```python
from build123d import *

# Parameters (mm, degrees)
SCHIZZO1_W                               = 70
SCHIZZO1_H                               = 100
ESTRUSIONE_ESTRUSIONE1_DEPTH             = 20
FORO_SVASATO_PER_VITE_M3_5_2_D           = 3.9
FORO_SVASATO_PER_VITE_M3_5_2_CSINK_D     = 8.2
FORO_SVASATO_PER_VITE_M3_5_2_CSINK_ANGLE = 90
SCHIZZO8_W                               = 85
SCHIZZO8_H                               = 40
TAGLIO_ESTRUSIONE1_DEPTH                 = 65.226162893
RACCORDO2_R                              = 5


with BuildPart() as part:
    # Schizzo1 → Estrusione-Estrusione1 (new body)
    with BuildSketch(Plane(origin=(0, 0, 0), x_dir=(0, 1, 0), z_dir=(0, 0, 1))):
        Rectangle(SCHIZZO1_W, SCHIZZO1_H)
    extrude(amount=ESTRUSIONE_ESTRUSIONE1_DEPTH)

    # Foro svasato per Vite M3.5-2 (through all)
    with Locations(Plane.XY.offset(20)):
        with Locations((-45, -20), (30, -29)):
            foro_svasato_per_vite_m3_5_2 = CounterSinkHole(FORO_SVASATO_PER_VITE_M3_5_2_D / 2, FORO_SVASATO_PER_VITE_M3_5_2_CSINK_D / 2, counter_sink_angle=FORO_SVASATO_PER_VITE_M3_5_2_CSINK_ANGLE)

    # Specchia1: Foro svasato per Vite M3.5-2 across plane
    add(foro_svasato_per_vite_m3_5_2.mirror(Plane.ZX), mode=Mode.SUBTRACT)

    # Schizzo8 → Taglio-Estrusione1 (cut, through all)
    with BuildSketch(Plane.XY.offset(20)):
        with Locations((7.5, 0)):
            Rectangle(SCHIZZO8_W, SCHIZZO8_H)
    extrude(amount=-TAGLIO_ESTRUSIONE1_DEPTH, mode=Mode.SUBTRACT)

    # Raccordo2
    raccordo2_edges = [part.edges().sort_by_distance(p)[0] for p in [
        (50, 20, 10),
        (50, -20, 10),
        (-35, -20, 10),
        (-35, 20, 10),
        (50, 35, 10),
        (50, -35, 10),
        (-50, -35, 10),
        (-50, 35, 10),
    ]]
    fillet(raccordo2_edges, radius=RACCORDO2_R)


solid = part.part
```
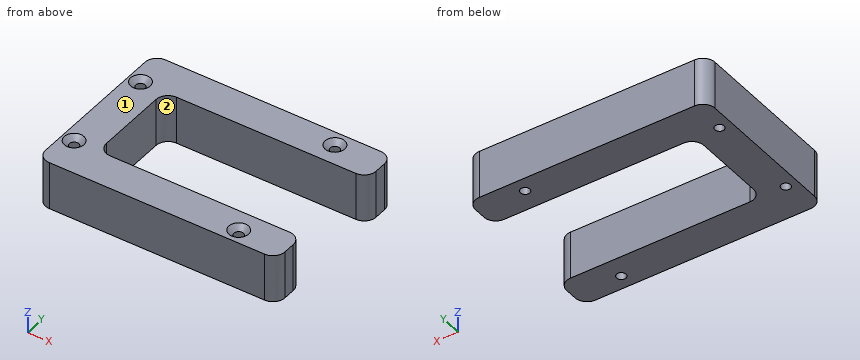
Design review of the part built by this model. Coordinates are the model's own, in mm. Face numbers are marked on the shaded views. A direction names the side the tool comes from. Give positions to 0.01 mm unless a question says otherwise; leave off trailing zeros. Loops run counter-clockwise (first coordinate to the right, second up) from the corner with the lowest first, then second, coordinate; pieces in that order, holes last. Notation, with made-up numbers: M -26,-21 L 20,-21 A12 cw 20,-12 Z; hole C 65,82 d4. An arc over 180 degrees is marked long. Return JSON: item names as keys, results as strings. Group by question number.
Item 1: Insertion check: pin 1 Ø5 at (x, y) = (21.5, -25.5) entering from -Z; pin 2 Ø12 at (y, z) = (1, 7) entering from +X; pin 3 Ø6 at (y, z) = (20.5, 18) entering from +X; pin 4 Ø2 at (y, z) = (-22, 5.5) entering from +X. Each pin has a flat end and moves straight along its axis. Give the tip position at first contact, or say it passes through.
Item 2: We need section C-C (z = 3.75). Give the boundary of the cut face in (x, y).
Item 3: For probe 1 along Y at (x, z) = (30, 11); probe 2 along Y at (x, z) = (39, 18); probe 3 along Y at (x, z) = (-45, 14), list the stretches that pass through material, from the lowest coordinate up.
Item 4: Tool access review of the marked faces 1 and 2: name each direction out of +Z, -Z, +X, -X, +Y, -Y from which nothing blocks a thin tool from reaching the whole face with its end or side.
Item 5: We need section D-D (x = 4.5). Give the boundary of the cut face in (y, z), and give its area (3 significant figures).
Item 6: We need section B-B (x = 30). Give the boundary of the cut face in (y, z), and give its area (3 significant figures).
Item 7: We need section A-A (y = -29). Give the boundary of the cut face in (x, z).
Output:
{
 "1": {"pin 1": "stops at z = 0", "pin 2": "stops at x = -35", "pin 3": "stops at x = 49.77", "pin 4": "stops at x = 49.58"},
 "2": {"outline": "M -50,-30 A5 ccw -45,-35 L 45,-35 A5 ccw 50,-30 L 50,-25 A5 ccw 45,-20 L -30,-20 A5 cw -35,-15 L -35,15 A5 cw -30,20 L 45,20 A5 ccw 50,25 L 50,30 A5 ccw 45,35 L -45,35 A5 ccw -50,30 Z; hole C -45,-20 d3.9; hole C -45,20 d3.9; hole C 30,-29 d3.9; hole C 30,29 d3.9"},
 "3": {"probe 1": "y = -35 to -30.95, -27.05 to -20, 20 to 27.05, 30.95 to 35", "probe 2": "y = -35 to -20, 20 to 35", "probe 3": "y = -35 to -21.95, -18.05 to 18.05, 21.95 to 35"},
 "4": {"face 1": "+Z, +X, -X, +Y, -Y", "face 2": "+Z, -Z, +X"},
 "5": {"outline": "M -35,0 L -20,0 L -20,20 L -35,20 Z; M 20,0 L 35,0 L 35,20 L 20,20 Z", "area": "600 mm^2"},
 "6": {"outline": "M -35,0 L -30.95,0 L -30.95,17.85 L -33.1,20 L -35,20 Z; M -27.05,0 L -20,0 L -20,20 L -24.9,20 L -27.05,17.85 Z; M 20,0 L 27.05,0 L 27.05,17.85 L 24.9,20 L 20,20 Z; M 30.95,0 L 35,0 L 35,20 L 33.1,20 L 30.95,17.85 Z", "area": "435 mm^2"},
 "7": {"outline": "M -50,0 L 28.05,0 L 28.05,17.85 L 25.9,20 L -50,20 Z; M 31.95,0 L 50,0 L 50,20 L 34.1,20 L 31.95,17.85 Z"}
}
